Check sheet for the drawn part. Datum: minimum x, y, z corner. Units: mm. Coordinates: 2 decimals unless noted, no trailing zeros. Order: outer loops, then holes, each group sorted by start corner. A loop starts at its lowest first (then second) coordinate and runs counter-clockwise, first axis right, second up.
1. Cross-section at A-A (x = 20). Count the separate pieces of the cut face and the enclosed holes in it, then the cut area to 3 significant figures.
2. Cross-section at C-C (z = 16.5). Enter the section's corners in (x, y), then the cut area to 3 significant figures.
3. Draft check along X on the marked faces 1 and 2. Enter one of: released by +X, released by -X, zero draft, split by the parting line, or undercut.
4. Gauge pin test, flat ends, axial feed: pin 1 Ø6 at (x, z) = (19.5, 12.5) entering from -Y; pin 2 Ø4.5 at (x, z) = (20, 10) entering from +Y (1 decimal); pin 3 Ø5 at (y, z) = (24, 21.5) entering from -X. Record the tip position at first contact, or that the pin passes through.
5. Cross-section at D-D (z = 10). Enter the section's corners in (x, y).
6. Thickness scan on line 1 (Z direction, x = 27.5, y = 38.5); line 2 (Y direction, x = 20, z = 9.5); line 3 (Z direction, x = 30, y = 9.5). Record the ranges inside material, lowest first.
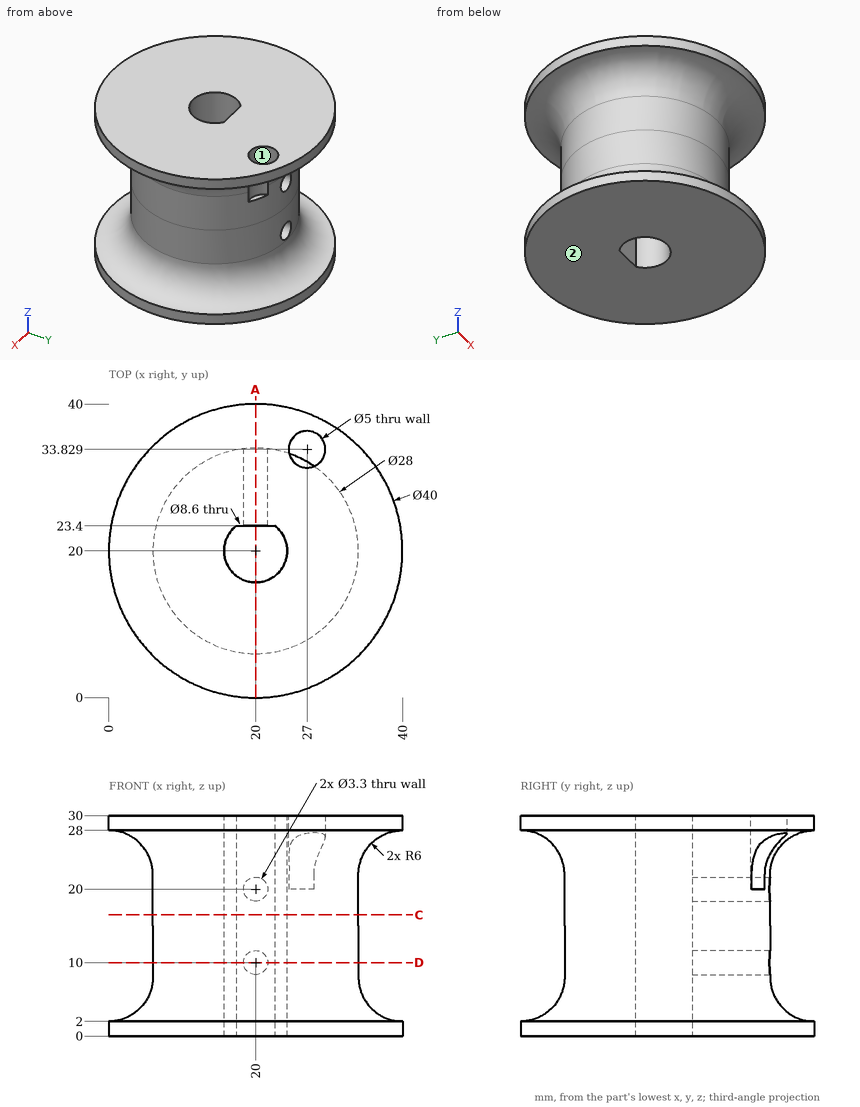
Data:
1. separate pieces: 4
1. enclosed holes: 0
1. area: 618 mm2
2. outline: circle Ø28 at (20, 20); hole (17.37, 23.4) arc R4.3 ccw (long way) to (22.63, 23.4) - close
2. area: 561 mm2
3. face 1: undercut
3. face 2: zero draft
4. pin 1: stops at y = 6
4. pin 2: stops at y = 34
4. pin 3: stops at x = 6.03
5. outline: (17.37, 23.4) - (18.35, 23.4) - (18.35, 33.9) arc R14 ccw (long way) to (21.65, 33.9) - (21.65, 23.4) - (22.63, 23.4) arc R4.3 cw (long way) to start
6. line 1: z = 0 to 2, 28 to 30
6. line 2: y = 6 to 15.7
6. line 3: z = 0 to 5.6, 24.4 to 30
